The model under review builds one solid part; all positions refer to its coordinate system, in mm. A direction names the side the tool comes from. Give positions to 0.01 mm unless a question says otherwise; leave off trailing zeros. Loops run counter-clockwise (first coordinate to the right, second up) from the corner with the lowest first, then second, coordinate; pieces in that order, holes last. Notation, with made-up numbers: (14.25, 9.5) - (55.25, 9.5) arc R13 cw to (55.25, 15.5) - close; hole circle Ø5 at (70.5, -36). An arc over 180 degrees is marked (long way). Answer as a JSON object with one key per item and string values.
from build123d import *

# Parameters (mm, degrees)
SKETCH1_R               = 20
BOSS_EXTRUDE1_DEPTH     = 15
CUT_EXTRUDE1_DEPTH      = 25
CUT_EXTRUDE1_DEPTH_BACK = 25
SKETCH2_W               = 15.2
SKETCH2_H               = 7.5
CUT_EXTRUDE2_REACH      = 34.016
SKETCH3_R               = 1.5
SKETCH4_R               = 2.6
CUT_EXTRUDE3_DEPTH      = 3


with BuildPart() as part:
    # Sketch1 → Boss-Extrude1 (new body)
    with BuildSketch(Plane(origin=(0, 0, 0), x_dir=(1, 0, 0), z_dir=(0, 1, 0))):
        with Locations(Location((0, 0, 0), (0, 0, 270))):
            Circle(SKETCH1_R)
    extrude(amount=BOSS_EXTRUDE1_DEPTH)

    # Sketch2 → Cut-Extrude1 (cut, two sides: drawn at the far end of the back side and taken through both)
    with BuildSketch(Plane.XY.offset(-CUT_EXTRUDE1_DEPTH_BACK)):
        with Locations((0, 3.75)):
            Rectangle(SKETCH2_W, SKETCH2_H)
    extrude(amount=CUT_EXTRUDE1_DEPTH + CUT_EXTRUDE1_DEPTH_BACK, mode=Mode.SUBTRACT)

    # Sketch3 → Cut-Extrude2 (cut, up to next)
    with BuildSketch(Plane(origin=(0, 0, 0), x_dir=(-1, 0, 0), z_dir=(0, -1, 0)), mode=Mode.PRIVATE) as cut_extrude2_sk1:
        with Locations(Location((14, -7, 0), (0, 0, 90))):
            Circle(SKETCH3_R)
    cut_extrude2_tool1 = extrude(cut_extrude2_sk1.sketch, amount=-CUT_EXTRUDE2_REACH, mode=Mode.PRIVATE) & part.part
    # Sketch3 → Cut-Extrude2 (cut, up to next)
    with BuildSketch(Plane(origin=(0, 0, 0), x_dir=(-1, 0, 0), z_dir=(0, -1, 0)), mode=Mode.PRIVATE) as cut_extrude2_sk2:
        with Locations(Location((14, 7, 0), (0, 0, 90))):
            Circle(SKETCH3_R)
    cut_extrude2_tool2 = extrude(cut_extrude2_sk2.sketch, amount=-CUT_EXTRUDE2_REACH, mode=Mode.PRIVATE) & part.part
    # Sketch3 → Cut-Extrude2 (cut, up to next)
    with BuildSketch(Plane(origin=(0, 0, 0), x_dir=(-1, 0, 0), z_dir=(0, -1, 0)), mode=Mode.PRIVATE) as cut_extrude2_sk3:
        with Locations(Location((-14, -7, 0), (0, 0, 90))):
            Circle(SKETCH3_R)
    cut_extrude2_tool3 = extrude(cut_extrude2_sk3.sketch, amount=-CUT_EXTRUDE2_REACH, mode=Mode.PRIVATE) & part.part
    # Sketch3 → Cut-Extrude2 (cut, up to next)
    with BuildSketch(Plane(origin=(0, 0, 0), x_dir=(-1, 0, 0), z_dir=(0, -1, 0)), mode=Mode.PRIVATE) as cut_extrude2_sk4:
        with Locations(Location((-14, 7, 0), (0, 0, 90))):
            Circle(SKETCH3_R)
    cut_extrude2_tool4 = extrude(cut_extrude2_sk4.sketch, amount=-CUT_EXTRUDE2_REACH, mode=Mode.PRIVATE) & part.part
    add(cut_extrude2_tool1.solids().sort_by_distance((-14, 0, 7))[0], mode=Mode.SUBTRACT)
    add(cut_extrude2_tool2.solids().sort_by_distance((-14, 0, -7))[0], mode=Mode.SUBTRACT)
    add(cut_extrude2_tool3.solids().sort_by_distance((14, 0, 7))[0], mode=Mode.SUBTRACT)
    add(cut_extrude2_tool4.solids().sort_by_distance((14, 0, -7))[0], mode=Mode.SUBTRACT)

    # Sketch4 → Cut-Extrude3 (cut)
    with BuildSketch(Plane(origin=(0, 15, 0), x_dir=(1, 0, 0), z_dir=(0, 1, 0))):
        with Locations(Location((-14, 7, 0), (0, 0, 270))):
            Circle(SKETCH4_R)
        with Locations(Location((-14, -7, 0), (0, 0, 270))):
            Circle(SKETCH4_R)
        with Locations(Location((14, 7, 0), (0, 0, 270))):
            Circle(SKETCH4_R)
        with Locations(Location((14, -7, 0), (0, 0, 270))):
            Circle(SKETCH4_R)
    extrude(amount=-CUT_EXTRUDE3_DEPTH, mode=Mode.SUBTRACT)


solid = part.part
Q1. Clearance check with flat-ended pins moving along their axes: pin 1 Ø8 at (x, y) = (11, 3.5) entering from -Z; pin 2 Ø5 at (y, z) = (7, 6) entering from -X; pin 3 Ø4 at (y, z) = (5, 4.5) entering from +X. State where each tip first meets the part, or that it passes through.
Results:
{"pin 1": "stops at z = -18.5", "pin 2": "stops at x = -19.69", "pin 3": "stops at x = 19.84"}
Q2. Consider section B-B, the plane y = 8.5. State the section outline as (x, z) points, plus the area to 3 significant figures.
Results:
{"outline": "circle Ø40 at (0, 0); hole circle Ø3 at (-14, -7); hole circle Ø3 at (-14, 7); hole circle Ø3 at (14, -7); hole circle Ø3 at (14, 7)", "area": "1,230 mm^2"}
Q3. To check wall thickness, follow probe 1 along X at (y, z) = (13.2, 7) (3 decimals); probe 2 along X at (y, z) = (9, 7) (3 decimals); probe 3 along Y at (x, z) = (3, -2). State the ranges of each line that lie inside material, in increasing order. Write a range as [from, to].
Results:
{"probe 1": "x = [-18.735, -16.6], [-11.4, 11.4], [16.6, 18.735]", "probe 2": "x = [-18.735, -15.5], [-12.5, 12.5], [15.5, 18.735]", "probe 3": "y = [7.5, 15]"}
Q4. Consider section C-C, the plane z = 0. State the section outline as (x, y) points.
Results:
{"outline": "(-20, 0) - (-7.6, 0) - (-7.6, 7.5) - (7.6, 7.5) - (7.6, 0) - (20, 0) - (20, 15) - (-20, 15) - close"}
Q5. For faces 5 (the face through (-16, 12, 7)), 6 (the face through (14.07, 5.92, 8.5)), 7 (the face through (0, 7.5, 0)), list the 3-axis set-ups (+Z, -Z, +X, -X, +Y, -Y) from which the entire face can be reached by the end or side of a thin tool; tool diameter is ignored.
Results:
{"face 5": "+Y", "face 6": "+Y, -Y", "face 7": "+Z, -Z, -Y"}
Q6. Consider section A-A, the plane x = 14. State the section outline as (y, z) points, plus the area to 3 significant figures.
Results:
{"outline": "(0, -14.28) - (15, -14.28) - (15, -9.6) - (12, -9.6) - (12, -8.5) - (0, -8.5) - close; (0, -5.5) - (12, -5.5) - (12, -4.4) - (15, -4.4) - (15, 4.4) - (12, 4.4) - (12, 5.5) - (0, 5.5) - close; (0, 8.5) - (12, 8.5) - (12, 9.6) - (15, 9.6) - (15, 14.28) - (0, 14.28) - close", "area": "325 mm^2"}
Q7. Consider section D-D, the plane z = 7. State the section outline as (x, y) points (3 decimals).
Results:
{"outline": "(-18.735, 0) - (-15.5, 0) - (-15.5, 12) - (-16.6, 12) - (-16.6, 15) - (-18.735, 15) - close; (-12.5, 0) - (-7.6, 0) - (-7.6, 7.5) - (7.6, 7.5) - (7.6, 0) - (12.5, 0) - (12.5, 12) - (11.4, 12) - (11.4, 15) - (-11.4, 15) - (-11.4, 12) - (-12.5, 12) - close; (15.5, 0) - (18.735, 0) - (18.735, 15) - (16.6, 15) - (16.6, 12) - (15.5, 12) - close"}
Q8. The part is to be moulded in two halves that separate along X. For faces 1 (the face through (-16, 12, -7)), 2 (the face through (7.6, 4, 0)), 3 (the face through (-12, 0, 0)), 4 (the face through (-19.524, 7.395, -4.336)), say which applies: +X half, -X half, draft (parallel to the pull), parting line (faces both ways), or undercut.
Results:
{"face 1": "undercut", "face 2": "undercut", "face 3": "draft", "face 4": "parting line"}
